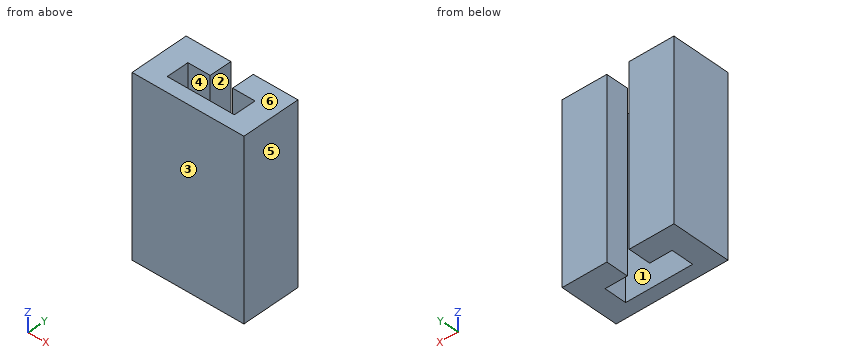
Autodesk Inventor part; units mm, degrees
ref_plane "YZ Plane" through (0, 0, 0) normal (1, 0, 0) x (0, 1, 0)
ref_plane "XZ Plane" through (0, 0, 0) normal (0, 1, 0) x (-1, 0, 0)
ref_plane "XY Plane" through (0, 0, 0) normal (0, 0, 1) x (1, 0, 0)
sketch "Sketch1" plane through (0, 0, 0) normal (0, 1, 0) x (-1, 0, 0)
  line L0 (0, 0) -> (16, 0)
  line L1 (16, 0) -> (16, -25.2)
  line L2 (16, -25.2) -> (0, -25.2)
  line L3 (0, -25.2) -> (0, 0)
  dimension "d0" = 16
  dimension "d1" = 25.2
extrude "Extrusion1" add sketch "Sketch1" along normal blind 2
sketch "Sketch2" plane through (-16, 0, 0) normal (0, 0, 1) x (1, 0, 0)
  line L0 (0, 2) -> (16, 2)
  line L1 (16, 2) -> (16, 8.4)
  line L2 (16, 8.4) -> (9.6, 8.4)
  line L3 (9.6, 8.4) -> (9.6, 5.2)
  line L4 (9.6, 5.2) -> (12.8, 5.2)
  line L5 (12.8, 5.2) -> (12.8, 2)
  line L6 (12.8, 2) -> (16, 2)
  line L7 (0, 2) -> (0, 8.4)
  line L8 (0, 8.4) -> (6.4, 8.4)
  line L9 (6.4, 8.4) -> (6.4, 5.2)
  line L10 (6.4, 5.2) -> (3.2, 5.2)
  line L11 (3.2, 5.2) -> (3.2, 2)
  point P0 (16, 0)
  dimension "d4" = 6.4
  dimension "d5" = 6.4
  dimension "d6" = 3.2
  dimension "d7" = 3.2
  dimension "d8" = 6.4
  dimension "d9" = 3.2
extrude "Extrusion2" add sketch "Sketch2" against normal blind 25.2
properties part number "testrail"
Can you work these out from the model? Positions are in its coordinate system, mm. Face numbers are marked on the shaded views. A direction names the side the tool comes from. Give positions to 0.01 mm unless a question says otherwise; leave off trailing zeros. Write each loop counter-clockwise with the first axis right and the second up, starting at its lowest first coordinate (ties: lowest second). Pieces come first, ordered by that corner, then holes. Notation, with made-up numbers: (88, 50) -> (109, 50) arc R35 cw to (109, 86) -> close; hole circle Ø4 at (-36.75, -5.5). An arc over 180 degrees is marked (long way). Answer as a JSON object with one key per item and string values. Group by question number.
Item 1: Suppose I cut it at A-A (y = 4). Please give me the cut outline in (x, z), plus the area to 3 significant figures.
Item 2: Suppose I cut it at C-C (z = -11.75). Please give me the cut outline in (x, y), plus the area to 3 significant figures.
Item 3: We'd pull the mould along X, two halves only. Please class the marked faces 4, 5 and 6: +X half, -X half, draft (parallel to the pull), parting line (faces both ways), or undercut.
Item 4: I'm going to push a flat-ended pin straight in: P1, Ø1, axis at x = -9.5, z = -8, coming from the +Y side. Where does the tip first touch, or does it pass through?
Item 5: Suppose I cut it at D-D (x = -7.5). Please give me the cut outline in (y, z), plus the area to 3 significant figures.
Item 6: Suppose I cut it at B-B (x = -10.5). Please give me the cut outline in (y, z).
Item 7: For the marked faces 1, 2 and 3, which set-ups out of +Z, -Z, +X, -X, +Y, -Y let a thin tool reach every point of the face, with its end or its side?
Item 8: Please list where these lines run through material, in increasing order: line 1 (Y direction, x = -10.75, z = -9); line 2 (X direction, y = 7, z = -6.75); line 3 (X direction, y = 2.5, z = -10.75). Write a range as [from, to].
Findings:
{
 "1": {"outline": "(-16, -25.2) -> (-12.8, -25.2) -> (-12.8, 0) -> (-16, 0) -> close; (-3.2, -25.2) -> (0, -25.2) -> (0, 0) -> (-3.2, 0) -> close", "area": "161 mm²"},
 "2": {"outline": "(-16, 0) -> (0, 0) -> (0, 8.4) -> (-6.4, 8.4) -> (-6.4, 5.2) -> (-3.2, 5.2) -> (-3.2, 2) -> (-12.8, 2) -> (-12.8, 5.2) -> (-9.6, 5.2) -> (-9.6, 8.4) -> (-16, 8.4) -> close", "area": "93.4 mm²"},
 "3": {"face 4": "undercut", "face 5": "+X half", "face 6": "draft"},
 "4": {"P1": "stops at y = 8.4"},
 "5": {"outline": "(0, -25.2) -> (2, -25.2) -> (2, 0) -> (0, 0) -> close", "area": "50.4 mm²"},
 "6": {"outline": "(0, -25.2) -> (2, -25.2) -> (2, 0) -> (0, 0) -> close; (5.2, -25.2) -> (8.4, -25.2) -> (8.4, 0) -> (5.2, 0) -> close"},
 "7": {"face 1": "+Z, -Z", "face 2": "+Z, -Z, +Y", "face 3": "+Z, -Z, +X, -X, -Y"},
 "8": {"line 1": "y = [0, 2], [5.2, 8.4]", "line 2": "x = [-16, -9.6], [-6.4, 0]", "line 3": "x = [-16, -12.8], [-3.2, 0]"}
}
